Source: three-view drawing plus pictorial views. Frame: mm from the lowest corner of the part. A direction names the side the tool comes from. Give positions to 0.01 mm unless a question says otherwise; leave off trailing zeros. Order: outer loops, then holes, each group sorted by start corner. A loop starts at its lowest first (then second) coordinate and runs counter-clockwise, first axis right, second up.
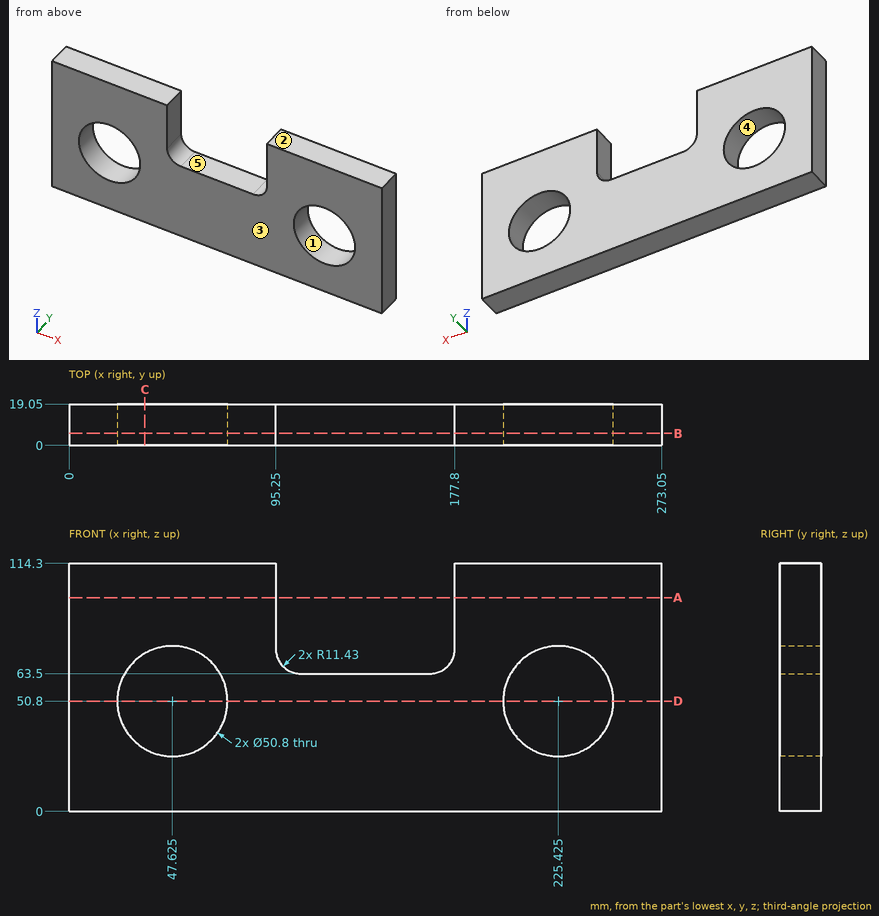
1) Section query B-B on y = 5.5. Output: boundary loops of the cut face in (x, z) (3 decimals), and give its area (3 significant figures).
Checks:
outline: (0, 0) - (273.05, 0) - (273.05, 114.3) - (177.8, 114.3) - (177.8, 74.93) arc R11.43 cw to (166.37, 63.5) - (106.68, 63.5) arc R11.43 cw to (95.25, 74.93) - (95.25, 114.3) - (0, 114.3) - close; hole circle Ø50.8 at (47.625, 50.8); hole circle Ø50.8 at (225.425, 50.8)
area: 23,000 mm2
2) First-contact query: pin 1 Ø9.5 at (x, y) = (123.5, 7.5) entering from +Z. Flat tip, straight axial feed; report the tip coordinate or a pass-through.
Checks:
pin 1: stops at z = 63.5
3) Section query C-C on x = 35. Output: boundary loops of the cut face in (y, z), and give its area (3 significant figures).
Checks:
outline: (0, 0) - (19.05, 0) - (19.05, 28.76) - (0, 28.76) - close; (0, 72.84) - (19.05, 72.84) - (19.05, 114.3) - (0, 114.3) - close
area: 1,340 mm2
4) Pull-direction query (Z, two-part tool) for the marked faces 1, 2 and 3; classes: +Z half, -Z half, draft (parallel to the pull), parting line (faces both ways), or undercut.
Checks:
face 1: undercut
face 2: +Z half
face 3: draft
5) Reachability of the marked faces 4 and 5 from +Z, -Z, +X, -X, +Y, -Y: full face, straight path, thin tool, end or side. Return the list, or none.
Checks:
face 4: +Y, -Y
face 5: +Z, +Y, -Y
6) Ray query, L1, parallel to X at y = 17.25, z = 49.5; L2, parallel to Z at x = 49, y = 9.5; L3, parallel to X at y = 12.25, z = 86.5. Return the intervals inside material, ascending.
Checks:
L1: x = 0 to 22.26, 72.99 to 200.06, 250.79 to 273.05
L2: z = 0 to 25.44, 76.16 to 114.3
L3: x = 0 to 95.25, 177.8 to 273.05
7) Section query D-D on z = 50.8. Output: boundary loops of the cut face in (x, y) (3 decimals), and give its area (3 significant figures).
Checks:
outline: (0, 0) - (22.225, 0) - (22.225, 19.05) - (0, 19.05) - close; (73.025, 0) - (200.025, 0) - (200.025, 19.05) - (73.025, 19.05) - close; (250.825, 0) - (273.05, 0) - (273.05, 19.05) - (250.825, 19.05) - close
area: 3,270 mm2
8) Section query A-A on z = 98.5. Output: boundary loops of the cut face in (x, y), and give its area (3 significant figures).
Checks:
outline: (0, 0) - (95.25, 0) - (95.25, 19.05) - (0, 19.05) - close; (177.8, 0) - (273.05, 0) - (273.05, 19.05) - (177.8, 19.05) - close
area: 3,630 mm2
